CAD build for the part. Positions are in the model's coordinates, mm. Face numbers are marked on the shaded views. Coordinates: 2 decimals unless noted, no trailing zeros. Write each loop counter-clockwise with the first axis right and the second up, starting at its lowest first coordinate (ties: lowest second). Pieces come first, ordered by that corner, then holes. Notation, with made-up numbers: (84.25, 6) - (140.25, 6) arc R32 cw to (140.25, 43) - close; hole circle Ø4 at (-15, -18). An arc over 180 degrees is marked (long way). Answer in a Markdown table with one row per item. Add a question column.
Q1. Band-saw the part on D-D (z = 17). List the corners of the cut face in (x, y), and give its area (3 significant figures).
Q2. Band-saw the part on B-B (x = 0). List the corners of the cut face in (y, z), and give its area (3 significant figures).
Q3. Pin check, flat tips, straight feed: pin 1 (1.5 mm diameter, centred on x = 24, y = 3.5, fed in from -Z); pin 2 (1.5 mm diameter, centred on x = -14.5, y = 1.5, fed in from +Z); pin 3 (1.5 mm diameter, centred on x = 32.5, y = 6, fed in from -Z). Stop position of each tip, or through.
Q4. Two-plate mould, pull along Z, no slides. Class the marked faces 1, 2 and 3: +Z half, -Z half, draft (parallel to the pull), parting line (faces both ways), or undercut.
Q5. Band-saw the part on C-C (y = 1.25). List the corners of the cut face in (x, z).
Q6. Drill centre lines: line 1 along X through (y, z) = (3.75, -4); line 2 along Z through (x, y) = (-24, 0.75); line 3 along Z through (x, y) = (11, 3). Where is each one in solid material? Low to high. Write a range as from..to.
Q7. Band-saw the part on A-A (z = 0). List the corners of the cut face in (x, y).
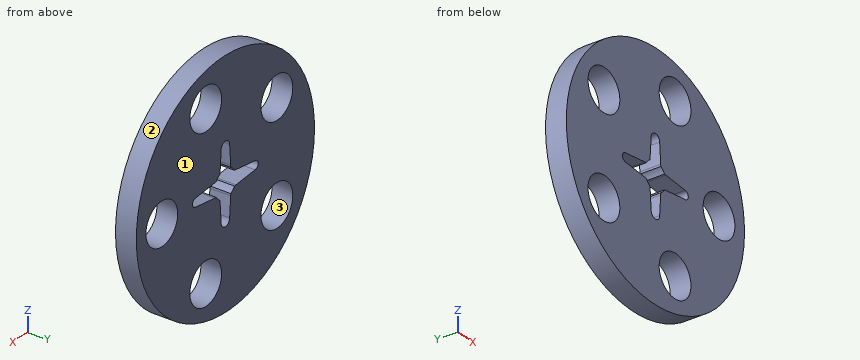
```python
from build123d import *

# Parameters (mm, degrees)
SKETCH1_R           = 42
SKETCH1_R_2         = 7.5
BOSS_EXTRUDE2_DEPTH = 7.5


with BuildPart() as part:
    # Sketch1 → Boss-Extrude2 (new body)
    with BuildSketch(Plane(origin=(0, 0, 0), x_dir=(1, 0, 0), z_dir=(0, 1, 0))):
        with Locations(Location((0, 0, 0), (0, 0, 270))):
            Circle(SKETCH1_R)
        with Locations(Location((30, 0, 0), (0, 0, 270))):
            Circle(SKETCH1_R_2, mode=Mode.SUBTRACT)
        with Locations(Location((9.270509831, -28.531695489, 0), (0, 0, 270))):
            Circle(SKETCH1_R_2, mode=Mode.SUBTRACT)
        with Locations(Location((-24.270509831, -17.633557569, 0), (0, 0, 270))):
            Circle(SKETCH1_R_2, mode=Mode.SUBTRACT)
        with Locations(Location((-24.270509831, 17.633557569, 0), (0, 0, 270))):
            Circle(SKETCH1_R_2, mode=Mode.SUBTRACT)
        with Locations(Location((9.270509831, 28.531695489, 0), (0, 0, 270))):
            Circle(SKETCH1_R_2, mode=Mode.SUBTRACT)
        with BuildLine():
            Line((4.999698513, -2.497254635), (4.285172416, -2.575710114))
            ThreePointArc((4.285172416, -2.575710114), (3.523319938, -3.547280908), (2.546607961, -4.302531013))
            Line((2.546607961, -4.302531013), (2.497527986, -4.99999802))
            Line((2.497527986, -4.99999802), (2, -12))
            ThreePointArc((2, -12), (0, -14), (-2, -12))
            Line((-2, -12), (-2.496981283, -4.99999802))
            Line((-2.496981283, -4.99999802), (-2.546494806, -4.302597986))
            ThreePointArc((-2.546494806, -4.302597986), (-3.523273292, -3.547327238), (-4.285172416, -2.575710114))
            Line((-4.285172416, -2.575710114), (-4.999698513, -2.497254635))
            Line((-4.999698513, -2.497254635), (-14, -1.5))
            ThreePointArc((-14, -1.5), (-15.5, 0), (-14, 1.5))
            Line((-14, 1.5), (-4.999698513, 2.497254635))
            Line((-4.999698513, 2.497254635), (-4.285172416, 2.575710114))
            ThreePointArc((-4.285172416, 2.575710114), (-3.523273292, 3.547327238), (-2.546494806, 4.302597986))
            Line((-2.546494806, 4.302597986), (-2.496981283, 4.99999802))
            Line((-2.496981283, 4.99999802), (-2, 12))
            ThreePointArc((-2, 12), (0, 14), (2, 12))
            Line((2, 12), (2.497527986, 4.99999802))
            Line((2.497527986, 4.99999802), (2.546607961, 4.302531013))
            ThreePointArc((2.546607961, 4.302531013), (3.523319938, 3.547280908), (4.285172416, 2.575710114))
            Line((4.285172416, 2.575710114), (4.999698513, 2.497254635))
            Line((4.999698513, 2.497254635), (14, 1.5))
            ThreePointArc((14, 1.5), (15.5, 0), (14, -1.5))
            Line((14, -1.5), (4.999698513, -2.497254635))
        make_face(mode=Mode.SUBTRACT)
    extrude(amount=BOSS_EXTRUDE2_DEPTH)


solid = part.part
```
Checked values:
| question | item | result |
|---|---|---|
| 1 | outline | (-38.41, 0) - (-31.74, 0) - (-31.74, 7.5) - (-38.41, 7.5) - close; (-16.8, 0) - (38.41, 0) - (38.41, 7.5) - (-16.8, 7.5) - close |
| 1 | area | 464 mm² |
| 2 | outline | (0, -42) - (7.5, -42) - (7.5, -14) - (0, -14) - close; (0, 14) - (7.5, 14) - (7.5, 42) - (0, 42) - close |
| 2 | area | 420 mm² |
| 3 | pin 1 | stops at z = -34.98 |
| 3 | pin 2 | stops at z = 39.69 |
| 3 | pin 3 | stops at z = -27.49 |
| 4 | face 1 | draft |
| 4 | face 2 | parting line |
| 4 | face 3 | undercut |
| 5 | outline | circle Ø84 at (0, 0); hole circle Ø15 at (-24.27, -17.63); hole circle Ø15 at (-24.27, 17.63); hole (-14, -1.5) - (-5, -2.5) - (-4.29, -2.58) arc R5 ccw to (-2.55, -4.3) - (-2, -12) arc R2 ccw to (2, -12) - (2.5, -5) - (2.55, -4.3) arc R5 ccw to (4.29, -2.58) - (5, -2.5) - (14, -1.5) arc R1.5 ccw to (14, 1.5) - (5, 2.5) - (4.29, 2.58) arc R5 ccw to (2.55, 4.3) - (2.5, 5) - (2, 12) arc R2 ccw to (-2, 12) - (-2.55, 4.3) arc R5 ccw to (-4.29, 2.58) - (-5, 2.5) - (-14, 1.5) arc R1.5 ccw to start; hole circle Ø15 at (9.27, -28.53); hole circle Ø15 at (9.27, 28.53); hole circle Ø15 at (30, 0) |
| 6 | line 1 | x = -41.81..-3, 3..23.66, 36.34..41.81 |
| 6 | line 2 | z = -34.47..-25.13, -10.14..10.14, 25.13..34.47 |
| 6 | line 3 | z = -40.53..-35.83, -21.23..-1.83, 1.83..21.23, 35.83..40.53 |
| 7 | outline | (-42, 0) - (-15.5, 0) - (-15.5, 7.5) - (-42, 7.5) - close; (15.5, 0) - (22.5, 0) - (22.5, 7.5) - (15.5, 7.5) - close; (37.5, 0) - (42, 0) - (42, 7.5) - (37.5, 7.5) - close |
